Geometry check sheet. Reference: the model listing, model coordinates, mm. Give positions to 0.01 mm unless a question says otherwise; leave off trailing zeros. Write each loop counter-clockwise with the first axis right and the second up, starting at its lowest first coordinate (ties: lowest second). Pieces come first, ordered by that corner, then holes. Notation, with made-up numbers: (16, 83) -> (75, 83) arc R15 cw to (75, 106) -> close; hole circle Ø4 at (79, 61.5). An arc over 180 degrees is marked (long way). One line per item, written item: value.
from build123d import *

# Parameters (mm, degrees)
BOSS_EXTRUDE1_DEPTH = 2.5
SKETCH2_R           = 2
CUT_EXTRUDE1_DEPTH  = 6


with BuildPart() as part:
    # Sketch1 → Boss-Extrude1 (new body, symmetric)
    with BuildSketch(Plane.XY):
        with BuildLine():
            Line((0, 4), (42, 4))
            ThreePointArc((42, 4), (46, 0), (42, -4))
            Line((42, -4), (0, -4))
            ThreePointArc((0, -4), (-4, 0), (0, 4))
        make_face()
    extrude(amount=BOSS_EXTRUDE1_DEPTH, both=True)

    # Sketch2 → Cut-Extrude1 (cut, through all)
    with BuildSketch(Plane.XY.offset(2.5)):
        with Locations((42, 0)):
            Circle(SKETCH2_R)
        Circle(SKETCH2_R)
    extrude(amount=-CUT_EXTRUDE1_DEPTH, mode=Mode.SUBTRACT)


solid = part.part
1) Sectioned sample at B-B on y = 0. Record the cut outline in (x, z), plus the area to 3 significant figures.
Verdict:
outline: (-4, -2.5) -> (-2, -2.5) -> (-2, 2.5) -> (-4, 2.5) -> close; (2, -2.5) -> (40, -2.5) -> (40, 2.5) -> (2, 2.5) -> close; (44, -2.5) -> (46, -2.5) -> (46, 2.5) -> (44, 2.5) -> close
area: 210 mm^2
2) Scan lines: probe 1 along Y at (x, z) = (0, -1.4); probe 2 along X at (y, z) = (-1, 0.45); probe 3 along X at (y, z) = (-1.75, -1.45). Record each from-to range of solid material in increasing order.
Verdict:
probe 1: -4 to -2, 2 to 4
probe 2: -3.87 to -1.73, 1.73 to 40.27, 43.73 to 45.87
probe 3: -3.6 to -0.97, 0.97 to 41.03, 42.97 to 45.6
3) Sectioned sample at A-A on z = -0.35. Record the cut outline in (x, y).
Verdict:
outline: (0, -4) -> (42, -4) arc R4 ccw to (42, 4) -> (0, 4) arc R4 ccw to start; hole circle Ø4 at (0, 0); hole circle Ø4 at (42, 0)
4) Mould release check, pull along Y, two halves, no side actions. Record for faces 1 (the cylindrical face through (40, 0, 0)), 2 (the flat face through (21, 0, -2.5)), 3 (the flat face through (21, -4, 0)): released by +Y, released by -Y, zero draft, split by the parting line, or undercut.
Verdict:
face 1: undercut
face 2: zero draft
face 3: released by -Y
5) Depth check by flat-ended pin: pin 1 Ø1 at (y, z) = (-2.5, 0.5) entering from +X; pin 2 Ø1 at (y, z) = (3, -1.5) entering from -X; pin 3 Ø3 at (y, z) = (-3, -0.5) entering from -X. Enter the tip coordinate at first touch or a pass-through.
Verdict:
pin 1: x = 45.46
pin 2: x = -3.12
pin 3: x = -3.71
